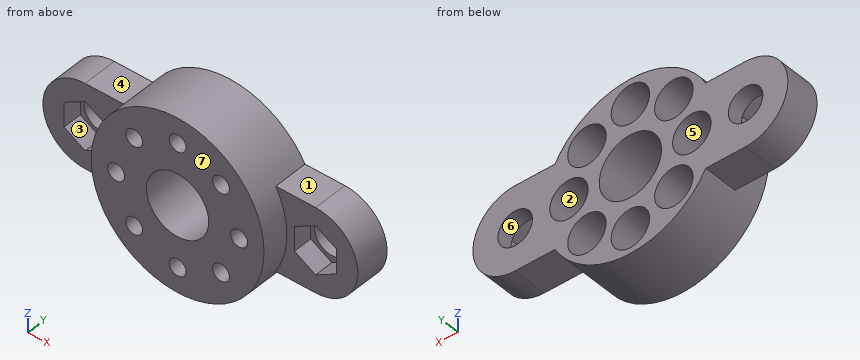
from build123d import *

# Parameters (mm, degrees)
SKETCH1_R           = 11.25
SKETCH1_R_2         = 1.1
SKETCH1_R_3         = 4.05
BOSS_EXTRUDE1_DEPTH = 8
SKETCH2_R           = 2.5
CUT_EXTRUDE1_DEPTH  = 6
SKETCH3_R           = 2.25
BOSS_EXTRUDE2_DEPTH = 4.5
CUT_EXTRUDE2_DEPTH  = 2.5


with BuildPart() as part:
    # Sketch1 → Boss-Extrude1 (new body)
    with BuildSketch(Plane(origin=(0, 0, 0), x_dir=(1, 0, 0), z_dir=(0, 1, 0))):
        Circle(SKETCH1_R)
        with Locations((0, 8)):
            Circle(SKETCH1_R_2, mode=Mode.SUBTRACT)
        with Locations((5.656854249, 5.656854249)):
            Circle(SKETCH1_R_2, mode=Mode.SUBTRACT)
        with Locations((8, 0)):
            Circle(SKETCH1_R_2, mode=Mode.SUBTRACT)
        with Locations((5.656854249, -5.656854249)):
            Circle(SKETCH1_R_2, mode=Mode.SUBTRACT)
        with Locations((0, -8)):
            Circle(SKETCH1_R_2, mode=Mode.SUBTRACT)
        with Locations((-5.656854249, -5.656854249)):
            Circle(SKETCH1_R_2, mode=Mode.SUBTRACT)
        with Locations((-8, 0)):
            Circle(SKETCH1_R_2, mode=Mode.SUBTRACT)
        with Locations((-5.656854249, 5.656854249)):
            Circle(SKETCH1_R_2, mode=Mode.SUBTRACT)
        Circle(SKETCH1_R_3, mode=Mode.SUBTRACT)
    extrude(amount=BOSS_EXTRUDE1_DEPTH)

    # Sketch2 → Cut-Extrude1 (cut)
    with BuildSketch(Plane(origin=(0, 8, 0), x_dir=(1, 0, 0), z_dir=(0, 1, 0))):
        with Locations((0, 8)):
            Circle(SKETCH2_R)
        with Locations((5.656854249, 5.656854249)):
            Circle(SKETCH2_R)
        with Locations((8, 0)):
            Circle(SKETCH2_R)
        with Locations((5.656854249, -5.656854249)):
            Circle(SKETCH2_R)
        with Locations((0, -8)):
            Circle(SKETCH2_R)
        with Locations((-5.656854249, -5.656854249)):
            Circle(SKETCH2_R)
        with Locations((-8, 0)):
            Circle(SKETCH2_R)
        with Locations((-5.656854249, 5.656854249)):
            Circle(SKETCH2_R)
    extrude(amount=-CUT_EXTRUDE1_DEPTH, mode=Mode.SUBTRACT)

    # Sketch3 → Boss-Extrude2 (add)
    with BuildSketch(Plane(origin=(0, 8, 0), x_dir=(1, 0, 0), z_dir=(0, 1, 0))):
        with BuildLine():
            Line((-15, 5.5), (-9.813893213, 5.5))
            ThreePointArc((-9.813893213, 5.5), (-11.25, 0), (-9.813893213, -5.5))
            Line((-9.813893213, -5.5), (-15, -5.5))
            ThreePointArc((-15, -5.5), (-20.5, 0), (-15, 5.5))
        make_face()
        with Locations((-15, 0)):
            Circle(SKETCH3_R, mode=Mode.SUBTRACT)
        with BuildLine():
            Line((9.813893213, 5.5), (15, 5.5))
            ThreePointArc((15, 5.5), (20.5, 0), (15, -5.5))
            Line((15, -5.5), (9.813893213, -5.5))
            ThreePointArc((9.813893213, -5.5), (11.25, 0), (9.813893213, 5.5))
        make_face()
        with Locations((15, 0)):
            Circle(SKETCH3_R, mode=Mode.SUBTRACT)
    extrude(amount=-BOSS_EXTRUDE2_DEPTH)

    # Sketch4 → Cut-Extrude2 (cut)
    with BuildSketch(Plane.XZ.offset(-3.5)):
        Polygon((-15, 3.175426481), (-17.75, 1.58771324), (-17.75, -1.58771324), (-15, -3.175426481), (-12.25, -1.58771324), (-12.25, 1.58771324), align=None)
        Polygon((12.25, 1.58771324), (15, 3.175426481), (17.75, 1.58771324), (17.75, -1.58771324), (15, -3.175426481), (12.25, -1.58771324), align=None)
    extrude(amount=-CUT_EXTRUDE2_DEPTH, mode=Mode.SUBTRACT)


solid = part.part
Design review of the part built by this model. Coordinates are the model's own, in mm. Face numbers are marked on the shaded views. A direction names the side the tool comes from. Round coordinates to 2 decimals unless told otherwise and drop trailing zeros. Order: outer loops, then holes, each group sorted by start corner. A loop starts at its lowest first (then second) coordinate and runs counter-clockwise, first axis right, second up.
1) For L1, parallel to X at y = 6.5, z = 0; L2, parallel to X at y = 1.05, z = 0, list the stretches that pass through material, from the lowest coordinate up.
The answers:
L1: x = -20.5 to -17.25, -12.75 to -10.5, -5.5 to -4.05, 4.05 to 5.5, 10.5 to 12.75, 17.25 to 20.5
L2: x = -11.25 to -9.1, -6.9 to -4.05, 4.05 to 6.9, 9.1 to 11.25
2) Clearance check with flat-ended pins moving along their axes: pin 1 Ø3.5 at (x, z) = (5.66, -5.66) entering from +Y; pin 2 Ø2 at (x, y) = (11.5, 7) entering from +Z; pin 3 Ø6 at (x, z) = (-14, -7) entering from -Y. State where each tip first meets the part, or that it passes through.
The answers:
pin 1: stops at y = 2
pin 2: stops at z = 5.5
pin 3: stops at y = 3.5
3) Draft analysis for pull direction Z (two halves, no side actions). For the marked faces 4, 5, 6 and 7, state which applies: released by +Z, released by -Z, zero draft, split by the parting line, or undercut.
The answers:
face 4: released by +Z
face 5: undercut
face 6: undercut
face 7: zero draft
4) Consider section A-A (x = 6). State the section outline as (y, z) points.
The answers:
outline: (0, -9.52) - (8, -9.52) - (8, -8.13) - (2, -8.13) - (2, -6.7) - (0, -6.7) - close; (0, -4.61) - (2, -4.61) - (2, -3.18) - (8, -3.18) - (8, -1.5) - (2, -1.5) - (2, 1.5) - (8, 1.5) - (8, 3.18) - (2, 3.18) - (2, 4.61) - (0, 4.61) - close; (0, 6.7) - (2, 6.7) - (2, 8.13) - (8, 8.13) - (8, 9.52) - (0, 9.52) - close
5) Machinability: for the marked faces 1, 2 and 3, which of the approach directions +Z, -Z, +X, -X, +Y, -Y give a long, thin tool a straight path to every point of the face, cutting with its end or side? Answer none if there is none.
The answers:
face 1: +Z, +X, +Y, -Y
face 2: +Y
face 3: -Y
6) Consider section D-D (z = -5). State the section outline as (x, y) points, plus the area to 3 significant figures.
The answers:
outline: (-17.29, 3.5) - (-10.08, 3.5) - (-10.08, 0) - (-6.54, 0) - (-6.54, 2) - (-8.07, 2) - (-8.07, 8) - (-17.29, 8) - close; (-4.77, 0) - (4.77, 0) - (4.77, 2) - (3.24, 2) - (3.24, 8) - (-3.24, 8) - (-3.24, 2) - (-4.77, 2) - close; (6.54, 0) - (10.08, 0) - (10.08, 3.5) - (17.29, 3.5) - (17.29, 8) - (8.07, 8) - (8.07, 2) - (6.54, 2) - close
area: 161 mm2
7) Consider section B-B (y = 1.5). Count the separate pieces of the cut face and the enclosed holes in it, plus the area to 3 significant figures.
The answers:
separate pieces: 1
enclosed holes: 9
area: 316 mm2
8) Consider section C-C (x = 0). State the section outline as (y, z) points, plus the area to 3 significant figures.
The answers:
outline: (0, -11.25) - (8, -11.25) - (8, -10.5) - (2, -10.5) - (2, -9.1) - (0, -9.1) - close; (0, -6.9) - (2, -6.9) - (2, -5.5) - (8, -5.5) - (8, -4.05) - (0, -4.05) - close; (0, 4.05) - (8, 4.05) - (8, 5.5) - (2, 5.5) - (2, 6.9) - (0, 6.9) - close; (0, 9.1) - (2, 9.1) - (2, 10.5) - (8, 10.5) - (8, 11.25) - (0, 11.25) - close
area: 46.4 mm2
